Check sheet for the modelled part. Datum: model origin and axes. Units: mm. Face numbers are marked on the shaded views. Give positions to 0.01 mm unless a question says otherwise; leave off trailing zeros. Order: outer loops, then holes, each group sorted by start corner. A loop starts at its lowest first (then second) coordinate and runs counter-clockwise, first axis right, second up. Notation, with made-up numbers: (73, -16) - (119, -16) arc R30 cw to (119, 15) - close; hole circle Ø9 at (35.25, 59). An arc over 180 degrees is marked (long way). Answer in a Markdown table with one row per item.
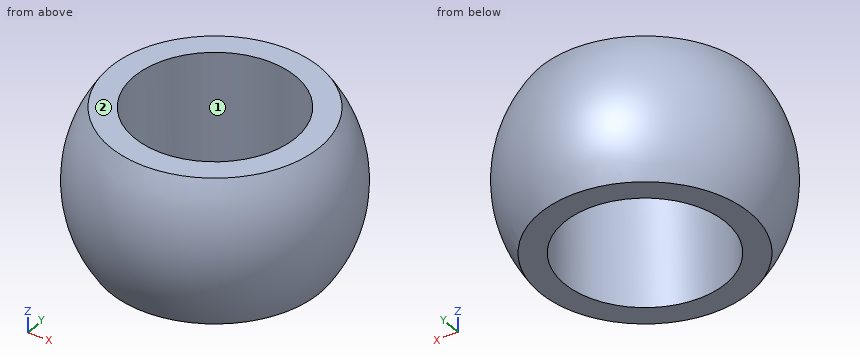
from build123d import *
from build123d.topology import SkipClean

# Parameters (mm, degrees)
CUT_EXTRUDE_1_DEPTH      = 10
CUT_EXTRUDE_1_DEPTH_BACK = 10
SKETCH_2_OUTSIDE_W       = 23.274
SKETCH_2_OUTSIDE_H       = 23.274
SKETCH_2_OUTSIDE_W_2     = 21.284245121
SKETCH_2_OUTSIDE_H_2     = 9
SKETCH_3_R               = 5
CUT_EXTRUDE_2_DEPTH      = 10


with BuildPart() as part:
    # Sketch 1 → Revolve 1 (revolve)
    with SkipClean():  # the faces are left unmerged after this step: merging them gives an invalid solid
        with BuildSketch(Plane(origin=(0, 0, 0), x_dir=(1, 0, 0), z_dir=(0, 1, 0))):
            with BuildLine():
                ThreePointArc((7.9, 0), (0, 7.9), (-7.9, 0))
                Line((-7.9, 0), (7.9, 0))
            make_face()
            with BuildLine():
                Line((7.9, 0), (-7.9, 0))
                ThreePointArc((-7.9, 0), (0, -7.9), (7.9, 0))
            make_face()
        revolve(axis=Axis((-7.9, 0, 0), (1, 0, 0)))
    add(part.part.scale(1), mode=Mode.REPLACE)  # the faces are merged on a copy

    # Sketch 2 outside → Cut-Extrude 1 (cut, two sides: drawn at the far end of the back side and taken through both)
    with BuildSketch(Plane(origin=(0, 0, 0), x_dir=(1, 0, 0), z_dir=(0, 1, 0)).offset(-CUT_EXTRUDE_1_DEPTH_BACK)):
        Rectangle(SKETCH_2_OUTSIDE_W, SKETCH_2_OUTSIDE_H)
        with Locations((-0.394714959, 0)):
            Rectangle(SKETCH_2_OUTSIDE_W_2, SKETCH_2_OUTSIDE_H_2, mode=Mode.SUBTRACT)
    extrude(amount=CUT_EXTRUDE_1_DEPTH + CUT_EXTRUDE_1_DEPTH_BACK, mode=Mode.SUBTRACT)

    # Sketch 3 → Cut-Extrude 2 (cut)
    with BuildSketch(Plane(origin=(0, 0, -4.5), x_dir=(-1, 0, 0), z_dir=(0, 0, -1))):
        Circle(SKETCH_3_R)
    extrude(amount=-CUT_EXTRUDE_2_DEPTH, mode=Mode.SUBTRACT)


solid = part.part
(1) Cross-section at D-D, the plane y = -5.75. Record the cut outline in (x, z), then the cut area to 3 significant figures.
Geometry says:
| item | result |
|---|---|
| outline | (-3.02, -4.5) - (3.02, -4.5) arc R5.42 ccw to (3.02, 4.5) - (-3.02, 4.5) arc R5.42 ccw to start |
| area | 84.7 mm² |
(2) Gauge pin test, flat ends, axial feed: P1, Ø1.5, axis at x = 6, z = -1.5, coming from the +Y side; P2, Ø1.5, axis at x = -1.5, z = -2, coming from the +Y side; P3, Ø2, axis at y = -3, z = -3, coming from the -X side; P4, Ø9, axis at x = 0, y = 0, coming from the +Z side. Record the tip position at first contact, or that the pin passes through.
Geometry says:
| item | result |
|---|---|
| P1 | y = 5.73 |
| P2 | y = 7.7 |
| P3 | x = -7.2 |
| P4 | through |
(3) Cross-section at A-A, the plane y = 0. Record the cut outline in (x, z), then the cut area to 3 significant figures.
Geometry says:
| item | result |
|---|---|
| outline | (-6.49, -4.5) - (-5, -4.5) - (-5, 4.5) - (-6.49, 4.5) arc R7.9 ccw to start; (5, -4.5) - (6.49, -4.5) arc R7.9 ccw to (6.49, 4.5) - (5, 4.5) - close |
| area | 44.1 mm² |
(4) Thickness scan on L1, parallel to X at y = 0.5, z = 3.25; L2, parallel to X at y = 2.5, z = 3.75; L3, parallel to Y at x = 0, z = 3.25. Record the ranges inside material, lowest first.
Geometry says:
| item | result |
|---|---|
| L1 | -7.18 to -4.97, 4.97 to 7.18 |
| L2 | -6.49 to -4.33, 4.33 to 6.49 |
| L3 | -7.2 to -5, 5 to 7.2 |
(5) Cross-section at C-C, the plane z = 1. Record the cut outline in (x, y).
Geometry says:
| item | result |
|---|---|
| outline | circle Ø15.67 at (0, 0); hole circle Ø10 at (0, 0) |
(6) Mould release check, pull along X, two halves, no side actions. Record for the marked faces 1 and 2: pulls with the +X half, pulls with the -X half, needs draft (parallel to the pull), parting line crosses it, or undercut.
Geometry says:
| item | result |
|---|---|
| face 1 | undercut |
| face 2 | needs draft |
